```python
from build123d import *

# Parameters (mm, degrees)
F0_R     = 103
F1_DEPTH = 36
F2_R     = 58
F3_DEPTH = 50
F4_R     = 58
F5_DEPTH = 15
F6_R     = 9.5
F7_DEPTH = 45
F8_W     = 6
F8_H     = 4
F9_DEPTH = 35
F10_R    = 2.9999


# Not quite as in the source:
# - a fillet or chamfer is up to 0.001 mm smaller than in the source, because OpenCascade refuses the exact size


with BuildPart() as f1:
    # F0 (on Right) → F1 (new body, symmetric)
    with BuildSketch(Plane.YZ):
        Circle(F0_R)
    extrude(amount=F1_DEPTH, both=True)

    # F2 (on face) → F3 (join)
    with BuildSketch(Plane.YZ.offset(36)):
        Circle(F2_R)
    extrude(amount=F3_DEPTH)

    # F4 (on face) → F5 (join)
    with BuildSketch(Plane(origin=(-36, 0, 0), x_dir=(0, -1, 0), z_dir=(-1, 0, 0))):
        Circle(F4_R)
    extrude(amount=F5_DEPTH)

    # F6 (on face) → F7 (join)
    with BuildSketch(Plane(origin=(-51, 0, 0), x_dir=(0, -1, 0), z_dir=(-1, 0, 0))):
        Circle(F6_R)
    extrude(amount=F7_DEPTH)

    # F8 (on face) → F9 (cut)
    with BuildSketch(Plane(origin=(-96, 0, 0), x_dir=(0, -1, 0), z_dir=(-1, 0, 0))):
        with Locations((0, 9.5)):
            Rectangle(F8_W, F8_H)
    extrude(amount=-F9_DEPTH, mode=Mode.SUBTRACT)

    # F10 (radius 3 in the source; OpenCascade refuses exactly that, so slightly less here)
    f10_edges = [f1.edges().sort_by_distance(p)[0] for p in [
        (-61, 3, 8.256939),
        (-61, -3, 8.256939),
    ]]
    fillet(f10_edges, radius=F10_R)


solid = f1.part
```
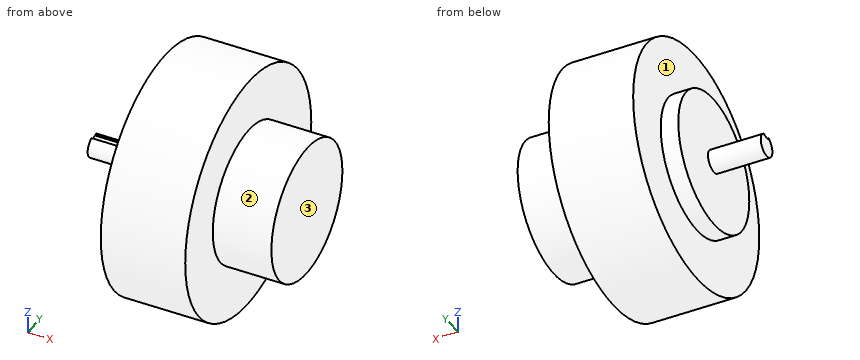
Here's how the part is built. I have some questions about the finished solid (model axes, mm). Face numbers are marked on the shaded views. A direction names the side the tool comes from. Coordinates: 2 decimals unless noted, no trailing zeros. Order: outer loops, then holes, each group sorted by start corner. A loop starts at its lowest first (then second) coordinate and runs counter-clockwise, first axis right, second up.
1) I need wall thicknesses on line 1 (X direction, y = 76.5, z = 27.5); line 2 (X direction, y = -35.5, z = -13.5); line 3 (Z direction, x = -21, y = 2). Which ranges of each line are inside material? Lowest first, please.
2) Will these pins go through, and if not, where does the flat tip stop? pin 1 (12 mm diameter, centred on y = -79, z = -20.5, fed in from -X); pin 2 (3 mm diameter, centred on x = -84.5, y = -0.5, fed in from +Z); pin 3 (1.5 mm diameter, centred on y = -35.5, z = -8, fed in from -X).
3) Imagine slicing it at A-A on z = 0. List the corners of the cut face in (x, y) for me, and give its area (3 significant figures).
4) Imagine slicing it at D-D on z = -53.5. List the corners of the cut face in (x, y) for me, and give its area (3 significant figures).
5) Imagine slicing it at C-C on x = 75.5. List the corners of the cut face in (y, z) for me, and give its area (3 significant figures).
6) Which directions (+Z, -Z, +X, -X, +Y, -Y) give clear straight access to the entire face, cutting with the end or side of a thin tool? Please do the marked faces 1, 2 and 3.
7) Imagine slicing it at B-B on y = -47.5. List the corners of the cut face in (x, z) for me, and give its area (3 significant figures).
Response values:
1. line 1: x = -36 to 36
1. line 2: x = -51 to 86
1. line 3: z = -102.98 to 102.98
2. pin 1: stops at x = -36
2. pin 2: stops at z = 7.5
2. pin 3: stops at x = -51
3. outline: (-96, -9.5) - (-51, -9.5) - (-51, -58) - (-36, -58) - (-36, -103) - (36, -103) - (36, -58) - (86, -58) - (86, 58) - (36, 58) - (36, 103) - (-36, 103) - (-36, 58) - (-51, 58) - (-51, 9.5) - (-96, 9.5) - close
3. area: 23,200 mm2
4. outline: (-51, -22.4) - (-36, -22.4) - (-36, -88.02) - (36, -88.02) - (36, -22.4) - (86, -22.4) - (86, 22.4) - (36, 22.4) - (36, 88.02) - (-36, 88.02) - (-36, 22.4) - (-51, 22.4) - close
4. area: 15,600 mm2
5. outline: circle Ø116 at (0, 0)
5. area: 10,600 mm2
6. face 1: -X
6. face 2: +X
6. face 3: +Z, -Z, +X, +Y, -Y
7. outline: (-51, -33.28) - (-36, -33.28) - (-36, -91.39) - (36, -91.39) - (36, -33.28) - (86, -33.28) - (86, 33.28) - (36, 33.28) - (36, 91.39) - (-36, 91.39) - (-36, 33.28) - (-51, 33.28) - close
7. area: 17,500 mm2
